The model under review builds one solid part; all positions refer to its coordinate system, in mm. Coordinates: 2 decimals unless noted, no trailing zeros. Order: outer loops, then holes, each group sorted by start corner. A loop starts at its lowest first (then second) coordinate and runs counter-clockwise, first axis right, second up. Notation, with made-up numbers: (5.5, 20.25) -> (29.5, 20.25) arc R27 cw to (29.5, 48.25) -> close; hole circle Ø7 at (-35.5, 4). An arc over 180 degrees is marked (long way). Use one line per item in the form item = value. Start each with the question number.
(1) Wall thickness on line 1 along Z through (x, y) = (58, 2.25); line 2 along X through (y, z) = (4.5, 1.2); line 3 along Y through (x, z) = (25, 2.1): over which ranges is each line inside the solid? List them lowest first.
(2) Insertion check: pin 1 Ø1 at (y, z) = (-3, 1.5) entering from +X; pin 2 Ø2 at (y, z) = (-1, 2) entering from +X; pin 3 Ø1.5 at (y, z) = (-3.5, 1) entering from -X; pin 4 Ø2 at (x, y) = (29, 1.5) entering from +Z. Each pin has a flat end and moves straight along its axis. Give the tip position at first contact, or say it passes through.
(3) Take a section at B-B (x = -50). State the section outline as (y, z) points.
(4) Take a section at A-A (y = 4.5). State the section outline as (x, z) points.
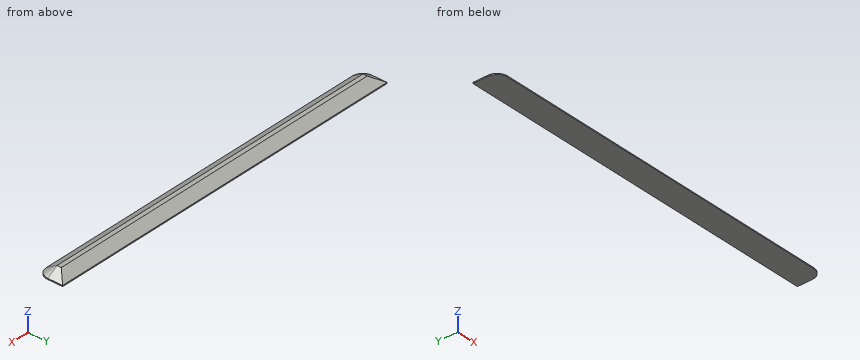
```python
from build123d import *

# Parameters (mm, degrees)
F1_DEPTH = 3.5
F2_SIZE2 = 2.99999
F2_SIZE  = 4.99999


# Not quite as in the source:
# - a fillet or chamfer is up to 0.001 mm smaller than in the source, because OpenCascade refuses the exact size


with BuildPart() as f1:
    # F0 (on Top) → F1 (new body)
    with BuildSketch(Plane.XY):
        with BuildLine():
            Line((-82.5, -6), (82.5, -6))
            ThreePointArc((82.5, -6), (86.0355339059, -4.5355339059), (87.5, -1))
            Line((87.5, -1), (87.5, 6))
            Line((87.5, 6), (-87.5, 6))
            Line((-87.5, 6), (-87.5, -1))
            ThreePointArc((-87.5, -1), (-86.0355339059, -4.5355339059), (-82.5, -6))
        make_face()
    extrude(amount=F1_DEPTH)

    # F2 (size 5 and 3 in the source; OpenCascade refuses exactly that, so slightly less here)
    f2_edges = [f1.edges().sort_by_distance(p)[0] for p in [
        (0, 6, 3.5),
        (87.5, 2.5, 3.5),
    ]]
    f2_side = f1.faces().sort_by_distance((0, 0.025079, 3.5))[0]
    chamfer(f2_edges, length=F2_SIZE, length2=F2_SIZE2, reference=f2_side)


solid = f1.part
```
Findings:
q1.line_1 = 0 to 2.75
q1.line_2 = -86.33 to 86.33
q1.line_3 = -3.33 to 3.33
q2.pin_1 = 86.19
q2.pin_2 = 86.67
q2.pin_3 = -87.11
q2.pin_4 = 3.5
q3.outline = (-6, 0) -> (6, 0) -> (6, 0.5) -> (1, 3.5) -> (-1, 3.5) -> (-6, 0.5) -> close
q4.outline = (-87.5, 0) -> (87.5, 0) -> (87.5, 0.5) -> (86, 1.4) -> (-86, 1.4) -> (-87.5, 0.5) -> close
